```python
from build123d import *

# Parameters (mm, degrees)
SKETCH_W        = 60
SKETCH_H        = 60
PAD_DEPTH       = 10.15
SKETCH001_R     = 2.1
SKETCH001_R_2   = 3.2
POCKET_DEPTH    = 12
SKETCH002_R     = 4.2
POCKET001_DEPTH = 3.6
FILLET_R        = 4
CHAMFER_SIZE    = 0.4
CHAMFER001_SIZE = 0.4
CHAMFER002_SIZE = 0.6


with BuildPart() as part:
    # Sketch → Pad (new body)
    with BuildSketch(Plane.XY):
        with Locations((30, 30)):
            Rectangle(SKETCH_W, SKETCH_H)
    extrude(amount=PAD_DEPTH)

    # Sketch001 (on Face6 of Pad) → Pocket (cut)
    with BuildSketch(Plane.XY.offset(10.15)):
        with Locations((15, 35)):
            Circle(SKETCH001_R)
        with Locations((45, 35)):
            Circle(SKETCH001_R)
        with Locations((15, 25)):
            Circle(SKETCH001_R)
        with Locations((45, 25)):
            Circle(SKETCH001_R)
        with Locations((10, 50)):
            Circle(SKETCH001_R_2)
        with Locations((50, 50)):
            Circle(SKETCH001_R_2)
        with Locations((10, 10)):
            Circle(SKETCH001_R_2)
        with Locations((50, 10)):
            Circle(SKETCH001_R_2)
    extrude(amount=-POCKET_DEPTH, mode=Mode.SUBTRACT)

    # Sketch002 (on Face5 of Pocket) → Pocket001 (cut)
    with BuildSketch(Plane.XY.offset(10.15)):
        with Locations((15, 35)):
            Circle(SKETCH002_R)
        with Locations((45, 35)):
            Circle(SKETCH002_R)
        with Locations((45, 25)):
            Circle(SKETCH002_R)
        with Locations((15, 25)):
            Circle(SKETCH002_R)
    extrude(amount=-POCKET001_DEPTH, mode=Mode.SUBTRACT)

    # Fillet
    fillet_edges = [part.edges().sort_by_distance(p)[0] for p in [
        (60, 0, 5.075),
        (0, 0, 5.075),
        (0, 60, 5.075),
        (60, 60, 5.075),
    ]]
    fillet(fillet_edges, radius=FILLET_R)

    # Chamfer
    chamfer_edges = [part.edges().sort_by_distance(p)[0] for p in [
        (30, 60, 10.15),
        (1.171573, 58.828427, 10.15),
        (58.828427, 58.828427, 10.15),
        (0, 30, 10.15),
        (60, 30, 10.15),
        (1.171573, 1.171573, 10.15),
        (58.828427, 1.171573, 10.15),
        (30, 0, 10.15),
        (40.8, 35, 10.15),
        (46.8, 50, 10.15),
        (6.8, 50, 10.15),
        (10.8, 35, 10.15),
        (10.8, 25, 10.15),
        (40.8, 25, 10.15),
        (46.8, 10, 10.15),
        (6.8, 10, 10.15),
    ]]
    chamfer(chamfer_edges, length=CHAMFER_SIZE)

    # Chamfer001
    chamfer001_edges = [part.edges().sort_by_distance(p)[0] for p in [
        (42.9, 35, 6.55),
        (42.9, 25, 6.55),
        (12.9, 25, 6.55),
        (12.9, 35, 6.55),
    ]]
    chamfer(chamfer001_edges, length=CHAMFER001_SIZE)

    # Chamfer002
    chamfer002_edges = [part.edges().sort_by_distance(p)[0] for p in [
        (30, 60, 0),
        (1.171573, 58.828427, 0),
        (58.828427, 58.828427, 0),
        (0, 30, 0),
        (60, 30, 0),
        (1.171573, 1.171573, 0),
        (58.828427, 1.171573, 0),
        (30, 0, 0),
        (42.9, 25, 0),
        (42.9, 35, 0),
        (46.8, 50, 0),
        (6.8, 50, 0),
        (12.9, 25, 0),
        (12.9, 35, 0),
        (46.8, 10, 0),
        (6.8, 10, 0),
    ]]
    chamfer(chamfer002_edges, length=CHAMFER002_SIZE)


solid = part.part
```
Here's how the part is built. I have some questions about the finished solid (model axes, mm). A direction names the side the tool comes from. Give positions to 0.01 mm unless a question says otherwise; leave off trailing zeros. Loops run counter-clockwise (first coordinate to the right, second up) from the corner with the lowest first, then second, coordinate; pieces in that order, holes last. Notation, with made-up numbers: M 66,-24.75 L 94,-24.75 A16 cw 94,-13.75 Z; hole C -17,-14 d1. An arc over 180 degrees is marked long. Put each result on its own line as item: value. Start each with the question number.
(1) I want a section at A-A on z = 4.5. State how many separate pieces and enclosed holes the cut face has, then the cut area to 3 significant figures.
(2) I want a section at B-B on y = 50. Please give me the cut outline in (x, z), then the cut area to 3 significant figures.
(3) If we mould it in two halves opening along X, with no side actions, what happens to faces 1 (the cylindrical face through (58.797, 58.859, 5.239)), 2 (the cylindrical face through (1.141, 58.797, 5.239)), 3 (the cylindrical face through (14.54, 32.95, 3.41)), 4 (the flat face through (30, 60, 5))? For each: +X half, -X half, draft (parallel to the pull), parting line (faces both ways), or undercut.
(4) For faces 5 (the conical face through (1.5, 1.45, 0.17)), 6 (the cylindrical face through (10.804, 25.185, 8.172)), which set-ups out of +Z, -Z, +X, -X, +Y, -Y let a thin tool reach every point of the face, with its end or its side?
(5) I need wall thicknesses on line 1 along Y through (x, z) = (45, 8); line 2 along Y through (x, z) = (11.5, 9); line 3 along X through (y, z) = (52.5, 1.5). Which ranges of each line are inside material? Lowest first, please. Write a range as [from, to].
(6) Will these pins go through, and if not, where does the flat tip stop? pin 1 Ø2.5 at (x, y) = (46, 26) entering from +Z; pin 2 Ø5.5 at (x, y) = (15, 35) entering from -Z; pin 3 Ø5 at (x, y) = (45, 35) entering from -Z.
Answer block:
1. separate pieces: 1
1. enclosed holes: 8
1. area: 3,400 mm^2
2. outline: M 0,0.6 L 0.6,0 L 6.2,0 L 6.8,0.6 L 6.8,9.75 L 6.4,10.15 L 0.4,10.15 L 0,9.75 Z; M 13.2,0.6 L 13.8,0 L 46.2,0 L 46.8,0.6 L 46.8,9.75 L 46.4,10.15 L 13.6,10.15 L 13.2,9.75 Z; M 53.2,0.6 L 53.8,0 L 59.4,0 L 60,0.6 L 60,9.75 L 59.6,10.15 L 53.6,10.15 L 53.2,9.75 Z
2. area: 478 mm^2
3. face 1: +X half
3. face 2: -X half
3. face 3: undercut
3. face 4: draft
4. face 5: -Z, -X, -Y
4. face 6: +Z
5. line 1: [0, 20.8], [29.2, 30.8], [39.2, 60]
5. line 2: [0, 7.17], [12.83, 22.68], [27.32, 32.68], [37.32, 47.17], [52.83, 60]
5. line 3: [0, 8], [12, 48], [52, 60]
6. pin 1: z = 6.55
6. pin 2: z = 0
6. pin 3: z = 0.2
